Geometry check sheet. Reference: the model listing, model coordinates, mm. A direction names the side the tool comes from. Round coordinates to 2 decimals unless told otherwise and drop trailing zeros. Write each loop counter-clockwise with the first axis right and the second up, starting at its lowest first coordinate (ties: lowest second). Pieces come first, ordered by that corner, then holes. Notation, with made-up numbers: (19.5, 40.5) -> (26.5, 40.5) arc R15 cw to (26.5, 47.5) -> close; hole circle Ø6 at (19.5, 58). An arc over 180 degrees is marked (long way). Use a Markdown table: item, result.
Autodesk Inventor part; units mm, degrees
ref_plane "YZ Plane" through (0, 0, 0) normal (1, 0, 0) x (0, 1, 0)
ref_plane "XZ Plane" through (0, 0, 0) normal (0, 1, 0) x (-1, 0, 0)
ref_plane "XY Plane" through (0, 0, 0) normal (0, 0, 1) x (1, 0, 0)
sketch "Szkic1" plane through (0, 0, 0) normal (0, 0, 1) x (1, 0, 0)
  line L0 (0, 0) -> (0, 30)
  line L1 (0, 30) -> (-12.5, 30)
  line L2 (-12.5, 30) -> (-12.5, 10)
  line L3 (-12.5, 10) -> (-25, 10)
  line L4 (-25, 10) -> (-25, 0)
  line L5 (-25, 0) -> (0, 0)
revolve "Obrót1" add sketch "Szkic1" angle 360 about axis through (0, 0, 0) along (0, 1, 0)
fillet "Zaokrąglenie1" radius 5 1 edges at (12.5, 10, 0)
chamfer "Faza1" distance 1 angle 45 2 edges at (12.5, 30, 0) (25, 10, 0)
sketch "Szkic2" plane through (0, 0, 0) normal (0, -1, 0) x (1, 0, 0)
  point P0 (0, 0)
hole "Otwór1" at (0, 0, 0) direction (0, 1, 0) diameter 10.106 depth 20 tip angle 118
properties part number "Projekt elementy" material "Stal"
(1) Release check for a two-part mould opening along Z. For faces 4 (the face through (-11.923, 21.902, -3.755)), 5 (the face through (-0.857, 22.509, 0.19)), 6 (the face through (0, 30, 0)) record: +Z half, -Z half, draft (parallel to the pull), parting line (faces both ways), or undercut.
A:
| item | result |
|---|---|
| face 4 | parting line |
| face 5 | undercut |
| face 6 | draft |
(2) Gauge pin test, flat ends, axial feed: pin 1 Ø8 at (x, y) = (-19.5, 23) entering from +Z; pin 2 Ø1 at (x, y) = (7, 7) entering from +Z; pin 3 Ø2 at (y, z) = (27, -5.5) entering from +X; pin 4 Ø2 at (x, y) = (-7, 21) entering from -Z. Record the tip position at first contact, or that the pin passes through.
A:
| item | result |
|---|---|
| pin 1 | passes through |
| pin 2 | stops at z = 24.14 |
| pin 3 | stops at x = 11.66 |
| pin 4 | stops at z = -10.97 |
(3) Access from +Z, -Z, +X, -X, +Y, -Y to the whole of each face (thin tool, end or side, straight path). Record for faces 1 (the face through (-2, 10, -18)), 2 (the face through (0.3, 0, -5.2)), 3 (the face through (3.075, 10.14, 4.01)).
A:
| item | result |
|---|---|
| face 1 | +Y |
| face 2 | +Z, -Z, +X, -X, -Y |
| face 3 | -Y |
(4) Thickness scan on line 1 (Z direction, x = 0, y = 5); line 2 (Y direction, x = -10.5, z = 19.5); line 3 (Z direction, x = 0, y = 15). Record the ranges inside material, lowest first.
A:
| item | result |
|---|---|
| line 1 | z = -25 to -5.05, 5.05 to 25 |
| line 2 | y = 0 to 10 |
| line 3 | z = -12.5 to -5.05, 5.05 to 12.5 |
(5) Section check A-A on y = 25.25. Record the cut outline in (x, z).
A:
| item | result |
|---|---|
| outline | circle Ø25 at (0, 0) |
(6) Section check B-B on y = 14.25. Record the cut outline in (x, z), plus the area to 3 significant figures.
A:
| item | result |
|---|---|
| outline | circle Ø25.11 at (0, 0); hole circle Ø10.11 at (0, 0) |
| area | 415 mm2 |
